Autodesk Inventor part; units mm, degrees
ref_plane "YZ Plane" through (0, 0, 0) normal (1, 0, 0) x (0, 1, 0)
ref_plane "XZ Plane" through (0, 0, 0) normal (0, 1, 0) x (-1, 0, 0)
ref_plane "XY Plane" through (0, 0, 0) normal (0, 0, 1) x (1, 0, 0)
sketch "Sketch1" plane through (0, 0, 0) normal (0, 1, 0) x (-1, 0, 0)
  arc A0 (-10.133, 6.6732) -> (-10.133, -6.6732) centre (0, 0) ccw
  line L0 (-10.133, -6.6732) -> (-8.8803, -5.8482)
  line L1 (-8.8803, 5.8482) -> (-10.133, 6.6732)
  arc A1 (-8.8803, 5.8482) -> (-8.8803, -5.8482) centre (0, 0) ccw
  point P0 (-12.133, 0)
  dimension "d0" = 12.133
  dimension "d2" = 12.133
  dimension "d3" = 0
  dimension "d5" = 2
  dimension "d6" = 2
  dimension "d7" = 1.5
extrude "Extrusion1" add sketch "Sketch1" along normal blind 20
sketch "Sketch2" plane through (0, 20, 0) normal (0, 1, 0) x (1, 0, 0)
  arc A0 (8.8803, -5.8482) -> (8.8803, 5.8482) centre (0, 0) ccw
  arc A1 (9.0178, 5.6338) -> (8.9103, 5.8024) centre (8.9645, 5.7183) ccw
  line L0 (0, 0) -> (10, 0)
  line L1 (10.133, 6.6732) -> (8.8803, 5.8482)
  line L2 (0, 0) -> (16.8616, 10.7558)
  dimension "d11" = 0.1
  dimension "d12" = 10
  dimension "d13" = 33.367
  dimension "d14" = 20
  dimension "d15" = 0.834
extrude "Extrusion2" cut sketch "Sketch2" against normal through all
pattern_circular "Circular Pattern1" count 40 over 66.79 about axis through (0, -10, 0) along (0, -1, 0) of "Extrusion2"
equation "\"d0\" = r"
equation "\"d7\" = t"
equation "\"segment\" = 2"
equation "\"t\" = 1.5"
equation "\"r\" = 12.133"
properties part number "holder3_cushion" material "Steel, Mild"
Build history of the part. All positions in model axes, mm. Round coordinates to 2 decimals unless told otherwise and drop trailing zeros. Write each loop counter-clockwise with the first axis right and the second up, starting at its lowest first coordinate (ties: lowest second). Pieces come first, ordered by that corner, then holes. Notation, with made-up numbers: M 0,-18 L 13,-18 A8 ccw 13,-14 Z; hole C 64,-26 d11. An arc over 180 degrees is marked long. Answer in a Markdown table with one row per item.
1. Flat gauge pins, fed straight in: P1, Ø3, axis at y = 10, z = -3.5, coming from the +X side; P2, Ø1, axis at x = 9.5, y = 5, coming from the -Z side. Where does each tip first touch, or does it go through?
Geometry check:
| item | result |
|---|---|
| P1 | x = 11.97 |
| P2 | z = -6.59 |
2. Probe L1, parallel to X at y = 15.75, z = -2.5; L2, parallel to X at y = 4.75, z = 1.75; L3, parallel to Z at x = 10.8, y = 6.25. List the from-to ranges inside material, lowest first. Write a range as [from, to].
Geometry check:
| item | result |
|---|---|
| L1 | [10.43, 11.87] |
| L2 | [10.49, 12.01] |
| L3 | [-5.53, 5.53] |
3. Saw through at A-A (x = 11.55). List the corners of the cut face in (y, z).
Geometry check:
| item | result |
|---|---|
| outline | M 0,-3.72 L 20,-3.72 L 20,3.72 L 0,3.72 Z |
